Could you check a few things on this drawing? It's one solid part, dimensions in mm from its lowest x, y, z. Give positions to 0.01 mm unless a question says otherwise; leave off trailing zeros. Loops run counter-clockwise (first coordinate to the right, second up) from the corner with the lowest first, then second, coordinate; pieces in that order, holes last. Notation, with made-up numbers: (-18, -13.75) - (13, -13.75) arc R13 ccw to (13, 6.25) - close; hole circle Ø10 at (43, 85.5). An arc over 180 degrees is marked (long way). Use CSV: the item, a comma, the result in double quotes.
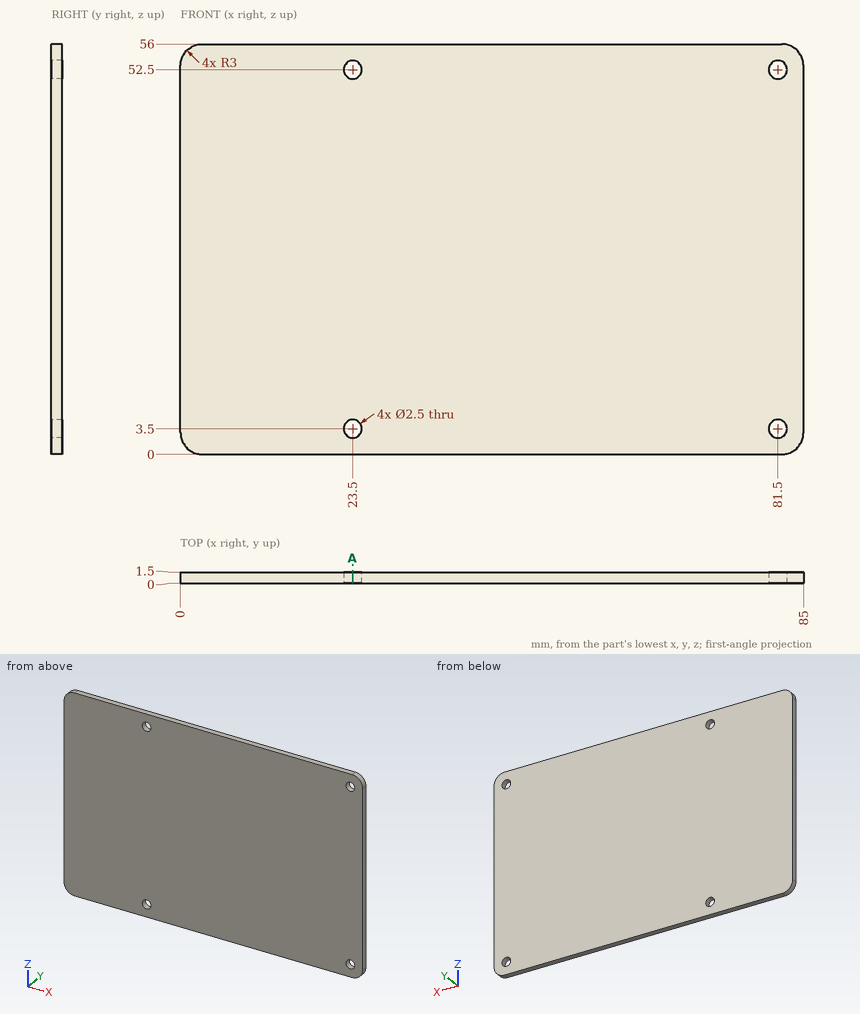
1) I need wall thicknesses on line 1 along Z through (x, y) = (23.5, 0.5); line 2 along X through (y, z) = (0.85, 52.5); line 3 along X through (y, z) = (0.95, 54). Which ranges of each line are inside material? Lowest first, please.
Answer below:
line 1,"z = 0 to 2.25, 4.75 to 51.25, 53.75 to 56"
line 2,"x = 0 to 22.25, 24.75 to 80.25, 82.75 to 85"
line 3,"x = 0.17 to 84.83"
2) Suppose I cut it at A-A (x = 23.5). Please give me the cut outline in (y, z).
Answer below:
outline,"(0, 0) - (1.5, 0) - (1.5, 2.25) - (0, 2.25) - close; (0, 4.75) - (1.5, 4.75) - (1.5, 51.25) - (0, 51.25) - close; (0, 53.75) - (1.5, 53.75) - (1.5, 56) - (0, 56) - close"
3) I'm going to push flat-ended pins straight in: P1, Ø4, axis at x = 23.5, z = 52.5, coming from the +Y side; P2, Ø2, axis at x = 81.5, z = 3.5, coming from the -Y side. Where does each tip first touch, or does it pass through?
Answer below:
P1,"stops at y = 1.5"
P2,"passes through"
